Read the model definition and answer for the solid it produces. Units are mm, in the model's axes. A direction names the side the tool comes from. Coordinates: 2 decimals unless noted, no trailing zeros. Order: outer loops, then holes, each group sorted by start corner. A loop starts at its lowest first (then second) coordinate and runs counter-clockwise, first axis right, second up.
```python
from build123d import *

# Parameters (mm, degrees)
BOSS_EXTRUDE1_DEPTH           = 15
CUT_EXTRUDE1_DEPTH            = 86.172406393
RIB1_REACH                    = 97.349
SKETCH4_WALL_W                = 257.512394394
SKETCH4_WALL_H                = 5
M3_CLEARANCE_HOLE1_AT_2_COUNT = 2
M3_CLEARANCE_HOLE1_AT_2_PITCH = 45
CUT_EXTRUDE2_DEPTH            = 3
FILLET1_R                     = 10


with BuildPart() as part:
    # Sketch1 → Boss-Extrude1 (new, symmetric)
    with BuildSketch(Plane.XY):
        Polygon((0, 0), (29.968527473, 74.174708365), (37.38599831, 71.177855618), (11.860487748, 8), (51.860487748, 8), (51.860487748, 0), align=None)
    extrude(amount=BOSS_EXTRUDE1_DEPTH, both=True)

    # Sketch2 → Cut-Extrude1 (cut, through all)
    with BuildSketch(Plane(origin=(0.379940125, 8, 0), x_dir=(1, 0, 0), z_dir=(0, 1, 0))):
        with BuildLine():
            Line((41.480547623, -3), (36.480547623, -3))
            ThreePointArc((36.480547623, -3), (33.480547623, 0), (36.480547623, 3))
            Line((36.480547623, 3), (41.480547623, 3))
            ThreePointArc((41.480547623, 3), (44.480547623, 0), (41.480547623, -3))
        make_face()
    extrude(amount=-CUT_EXTRUDE1_DEPTH, mode=Mode.SUBTRACT)

    # Sketch4 wall → Rib1 (add, up to next)
    with BuildSketch(Plane(origin=(44.623243029, 39.588927809, 15), x_dir=(0.223320905083, -0.974744978624, 0), z_dir=(0.974744978624, 0.223320905083, 0)), mode=Mode.PRIVATE) as rib1_sk1:
        with Locations((0, 2.5)):
            Rectangle(SKETCH4_WALL_W, SKETCH4_WALL_H)
    rib1_tool1 = extrude(rib1_sk1.sketch, amount=-RIB1_REACH, mode=Mode.PRIVATE) - part.part
    rib1 = rib1_tool1.solids().sort_by_distance((44.623243029, 39.588927809, 15))[0]
    add(rib1)

    # Mirror1: Rib1 across plane
    add(rib1.mirror(Plane.XY))

    # Sketch7 → M3 Clearance Hole1 (revolve, cut)
    with BuildSketch(Plane(origin=(33.639932376, 61.906017072, 0), x_dir=(0.37460659341591607, 0.9271838545667858, 0), z_dir=(0, 0, 1))):
        Polygon((0, 0), (0, 35.786334818), (1.7, 35.786334818), (1.7, 0.025), (1.725, 0), align=None)
    m3_clearance_hole1 = revolve(axis=Axis((39.527549852, 59.527265204, 0), (-0.9271838545667858, 0.37460659341591607, 0)), mode=Mode.SUBTRACT)

    # M3 Clearance Hole1 at 2: M3 Clearance Hole1 ×2
    with Locations(*[Vector(-0.37460659341591607, -0.9271838545667858, 0) * (i * M3_CLEARANCE_HOLE1_AT_2_PITCH) for i in range(1, M3_CLEARANCE_HOLE1_AT_2_COUNT)]):
        add(m3_clearance_hole1, mode=Mode.SUBTRACT)

    # Sketch8 → Cut-Extrude2 (cut)
    with BuildSketch(Plane(origin=(7.417470837, -2.996852747, 0), x_dir=(0, 0, -1), z_dir=(0.9271838545667858, -0.37460659341591607, 0))):
        Polygon((3.637306696, 70), (1.818653348, 73.15), (-1.818653348, 73.15), (-3.637306696, 70), (-1.818653348, 66.85), (1.818653348, 66.85), align=None)
        Polygon((3.637306696, 25), (1.818653348, 28.15), (-1.818653348, 28.15), (-3.637306696, 25), (-1.818653348, 21.85), (1.818653348, 21.85), align=None)
    extrude(amount=-CUT_EXTRUDE2_DEPTH, mode=Mode.SUBTRACT)

    # Fillet1
    # the kernel refuses this fillet: 10 mm, written as the material it adds along each edge
    with BuildSketch(Plane(origin=(11.860487748, 8, 47.064024213), x_dir=(0.3746065934159096, 0.9271838545667884, 0), z_dir=(0, 0, -1))) as fillet1_piece_1_section:
        with BuildLine():
            CenterArc((FILLET1_R * 1.48256096851, FILLET1_R), FILLET1_R, 158, 112)
            Line((FILLET1_R * 0.555377113946, FILLET1_R * 1.37460659342), (0, 0))
            Line((0, 0), (FILLET1_R * 1.48256096851, 0))
        make_face()
    fillet1_piece_1 = extrude(amount=94.128048426, mode=Mode.PRIVATE)
    fillet1_piece_1 = split(fillet1_piece_1, bisect_by=Plane(origin=(16.410561538, 18.315636212, 15), z_dir=(0, 0, -1)), keep=Keep.TOP, mode=Mode.PRIVATE)
    fillet1_piece_1 = split(fillet1_piece_1, bisect_by=Plane(origin=(17.191225171, 20.247846508, 3.760526332), z_dir=(-0.18730329670795798, -0.46359192728339266, 0.866025403784439)), keep=Keep.TOP, mode=Mode.PRIVATE)
    add(fillet1_piece_1)
    with BuildSketch(Plane(origin=(11.860487748, 8, 47.064024213), x_dir=(0.3746065934159096, 0.9271838545667884, 0), z_dir=(0, 0, -1))) as fillet1_piece_2_section:
        with BuildLine():
            CenterArc((FILLET1_R * 1.48256096851, FILLET1_R), FILLET1_R, 158, 112)
            Line((FILLET1_R * 0.555377113946, FILLET1_R * 1.37460659342), (0, 0))
            Line((0, 0), (FILLET1_R * 1.48256096851, 0))
        make_face()
    fillet1_piece_2 = extrude(amount=94.128048426, mode=Mode.PRIVATE)
    fillet1_piece_2 = split(fillet1_piece_2, bisect_by=Plane(origin=(16.998453552, 20.640654754, 3.929107959), z_dir=(0.18730329670795798, 0.46359192728339266, -0.866025403784439)), keep=Keep.TOP, mode=Mode.PRIVATE)
    fillet1_piece_2 = split(fillet1_piece_2, bisect_by=Plane(origin=(16.998453552, 20.640654754, 3.345505432), z_dir=(0.18730329670795837, 0.4635919272833937, 0.8660254037844384)), keep=Keep.TOP, mode=Mode.PRIVATE)
    add(fillet1_piece_2)
    with BuildSketch(Plane(origin=(11.860487748, 8, 47.064024213), x_dir=(0.3746065934159096, 0.9271838545667884, 0), z_dir=(0, 0, -1))) as fillet1_piece_3_section:
        with BuildLine():
            CenterArc((FILLET1_R * 1.48256096851, FILLET1_R), FILLET1_R, 158, 112)
            Line((FILLET1_R * 0.555377113946, FILLET1_R * 1.37460659342), (0, 0))
            Line((0, 0), (FILLET1_R * 1.48256096851, 0))
        make_face()
    fillet1_piece_3 = extrude(amount=57.064024213, mode=Mode.PRIVATE)
    fillet1_piece_3 = split(fillet1_piece_3, bisect_by=Plane(origin=(16.596548346, 16.860543337, 0), z_dir=(-0.3746065934159161, -0.9271838545667858, 0)), keep=Keep.TOP, mode=Mode.PRIVATE)
    fillet1_piece_3 = split(fillet1_piece_3, bisect_by=Plane(origin=(17.125135573, 18.168842634, 4.641292114), z_dir=(-0.18730329670795837, -0.4635919272833937, -0.8660254037844384)), keep=Keep.TOP, mode=Mode.PRIVATE)
    add(fillet1_piece_3)
    with BuildSketch(Plane(origin=(11.860487748, 8, 47.064024213), x_dir=(0.3746065934159096, 0.9271838545667884, 0), z_dir=(0, 0, -1))) as fillet1_piece_4_section:
        with BuildLine():
            CenterArc((FILLET1_R * 1.48256096851, FILLET1_R), FILLET1_R, 158, 112)
            Line((FILLET1_R * 0.555377113946, FILLET1_R * 1.37460659342), (0, 0))
            Line((0, 0), (FILLET1_R * 1.48256096851, 0))
        make_face()
    fillet1_piece_4 = extrude(amount=57.064024213, mode=Mode.PRIVATE)
    fillet1_piece_4 = split(fillet1_piece_4, bisect_by=Plane(origin=(16.526523366, 18.36657569, -2.60970235), z_dir=(-0.18730329670795812, -0.463591927283393, -0.8660254037844388)), keep=Keep.TOP, mode=Mode.PRIVATE)
    add(fillet1_piece_4)
    with BuildSketch(Plane(origin=(11.860487748, 8, 47.064024213), x_dir=(0.3746065934159096, 0.9271838545667884, 0), z_dir=(0, 0, -1))) as fillet1_piece_5_section:
        with BuildLine():
            CenterArc((FILLET1_R * 1.48256096851, FILLET1_R), FILLET1_R, 158, 112)
            Line((FILLET1_R * 0.555377113946, FILLET1_R * 1.37460659342), (0, 0))
            Line((0, 0), (FILLET1_R * 1.48256096851, 0))
        make_face()
    fillet1_piece_5 = extrude(amount=94.128048426, mode=Mode.PRIVATE)
    fillet1_piece_5 = split(fillet1_piece_5, bisect_by=Plane(origin=(16.998453552, 20.640654754, -3.929107959), z_dir=(0.18730329670795812, 0.463591927283393, 0.8660254037844388)), keep=Keep.TOP, mode=Mode.PRIVATE)
    fillet1_piece_5 = split(fillet1_piece_5, bisect_by=Plane(origin=(16.998453552, 20.640654754, -3.345505432), z_dir=(0.18730329670795812, 0.4635919272833931, -0.8660254037844387)), keep=Keep.TOP, mode=Mode.PRIVATE)
    add(fillet1_piece_5)


solid = part.part
```
1) Straight lines are drawn through the part: line 1 (Z direction, x = 19, y = 22.5); line 2 (Y direction, x = 46, z = -1); line 3 (Z direction, x = 36, y = 5). For each, find the intervals that lie inside material, in ascending order.
A:
line 1: z = -15 to -10, 10 to 15
line 2: y = 0 to 8
line 3: z = -15 to -2.87, 2.87 to 15
2) A cutting plane is placed at A-A, the plane z = -11. Determine the outline of the cut face in (x, y).
A:
outline: (0, 0) - (51.86, 0) - (51.86, 8) - (37.39, 71.18) - (29.97, 74.17) - close
3) Determine the mould class of faces 4 (the flat face through (26, 29, 15)), 5 (the flat face through (27, 26, -15)), 6 (the cylindrical face through (33.86, 4.06, 0.07)) for opening direction Z: pulls with the +Z half, pulls with the -Z half, needs draft (parallel to the pull), parting line crosses it, or undercut.
A:
face 4: pulls with the +Z half
face 5: pulls with the -Z half
face 6: undercut
4) A cutting plane is placed at D-D, the plane y = 35. Determine the outline of the cut face in (x, z).
A:
outline: (14.14, -15) - (45.67, -15) - (45.67, -10) - (22.77, -10) - (22.77, 10) - (45.67, 10) - (45.67, 15) - (14.14, 15) - close
5) A cutting plane is placed at C-C, the plane z = 0. Determine the outline of the cut face in (x, y), and give its area (3 significant figures).
A:
outline: (0, 0) - (33.86, 0) - (33.86, 8) - (26.69, 8) arc R10 cw to (16.76, 16.79) - (12.82, 18.39) - (13.36, 19.73) - (8.73, 21.6) - close; (10, 24.76) - (14.64, 22.88) - (15.18, 24.23) - (17.96, 23.1) - (32.46, 58.99) - (29.68, 60.11) - (30.22, 61.45) - (25.59, 63.33) - close; (26.86, 66.48) - (31.5, 64.61) - (32.04, 65.95) - (34.82, 64.83) - (37.39, 71.18) - (29.97, 74.17) - close; (44.86, 0) - (51.86, 0) - (51.86, 8) - (44.86, 8) - close
area: 849 mm2
6) Flat-ended cylindrical pins translate along their axes: pin 1 Ø8 at (y, z) = (41, -11) entering from +X; pin 2 Ø2 at (y, z) = (31.5, -11) entering from +X; pin 3 Ø1.5 at (x, z) = (15.5, -12) entering from +Y. Find the tip coordinate at first contact, or state that the pin passes through.
A:
pin 1: stops at x = 45.22
pin 2: stops at x = 46.71
pin 3: stops at y = 40.22
7) Which of the six approach directions +Z, -Z, +X, -X, +Y, -Y give full straight-line access (tool end or side, diameter ignored) to faces 1 (the flat face through (33.4, 65.4, 0)), 2 (the flat face through (27.54, 46.81, 0.14)), 3 (the flat face through (26, 0, 0))?
A:
face 1: none
face 2: +X
face 3: +Z, -Z, +X, -X, -Y
8) A cutting plane is placed at B-B, the plane x = 41. Determine the outline of the cut face in (y, z).
A:
outline: (0, -15) - (55.4, -15) - (55.4, -10) - (8, -10) - (8, -3) - (0, -3) - close; (0, 3) - (8, 3) - (8, 10) - (55.4, 10) - (55.4, 15) - (0, 15) - close
